```python
from build123d import *

# Parameters (mm, degrees)
BOSS_EXTRUDE1_DEPTH = 3.5
SKETCH2_R           = 3.55
BOSS_EXTRUDE2_DEPTH = 1
SKETCH3_W           = 2.85
SKETCH3_H           = 2.85
BOSS_EXTRUDE3_DEPTH = 1
SKETCH4_W           = 3.9
SKETCH4_H           = 3.9
SKETCH4_R           = 1
BOSS_EXTRUDE4_DEPTH = 2.15
SKETCH5_W           = 1
SKETCH5_H           = 1.5
BOSS_EXTRUDE5_DEPTH = 0.4


with BuildPart() as part:
    # Sketch1 → Boss-Extrude1 (new body)
    with BuildSketch(Plane(origin=(0, 0, 0), x_dir=(1, 0, 0), z_dir=(0, 1, 0))):
        with BuildLine():
            Line((-5, -6), (5, -6))
            ThreePointArc((5, -6), (5.707106781, -5.707106781), (6, -5))
            Line((6, -5), (6, 5))
            ThreePointArc((6, 5), (5.707106781, 5.707106781), (5, 6))
            Line((5, 6), (-5, 6))
            ThreePointArc((-5, 6), (-5.707106781, 5.707106781), (-6, 5))
            Line((-6, 5), (-6, -5))
            ThreePointArc((-6, -5), (-5.707106781, -5.707106781), (-5, -6))
        make_face()
    extrude(amount=BOSS_EXTRUDE1_DEPTH)

    # Sketch2 → Boss-Extrude2 (add)
    with BuildSketch(Plane(origin=(0, 3.5, 0), x_dir=(1, 0, 0), z_dir=(0, 1, 0))):
        with Locations(Location((0, 0, 0), (0, 0, 270))):
            Circle(SKETCH2_R)
    extrude(amount=BOSS_EXTRUDE2_DEPTH)

    # Sketch3 → Boss-Extrude3 (add)
    with BuildSketch(Plane(origin=(0, 4.5, 0), x_dir=(1, 0, 0), z_dir=(0, 1, 0))):
        Rectangle(SKETCH3_W, SKETCH3_H)
    extrude(amount=BOSS_EXTRUDE3_DEPTH)

    # Sketch4 → Boss-Extrude4 (add)
    with BuildSketch(Plane(origin=(0, 5.5, 0), x_dir=(1, 0, 0), z_dir=(0, 1, 0))):
        Rectangle(SKETCH4_W, SKETCH4_H)
        with Locations(Location((0, 0, 0), (0, 0, 90))):
            Circle(SKETCH4_R, mode=Mode.SUBTRACT)
    extrude(amount=BOSS_EXTRUDE4_DEPTH)

    # Sketch5 → Boss-Extrude5 (add)
    with BuildSketch(Plane.XY.offset(6)):
        with Locations((-2.547676789, 0)):
            Rectangle(SKETCH5_W, SKETCH5_H)
        with Locations((2.547676789, 0)):
            Rectangle(SKETCH5_W, SKETCH5_H)
    boss_extrude5 = extrude(amount=BOSS_EXTRUDE5_DEPTH)

    # Mirror1: Boss-Extrude5 across plane
    add(boss_extrude5.mirror(Plane.XY))


solid = part.part
```
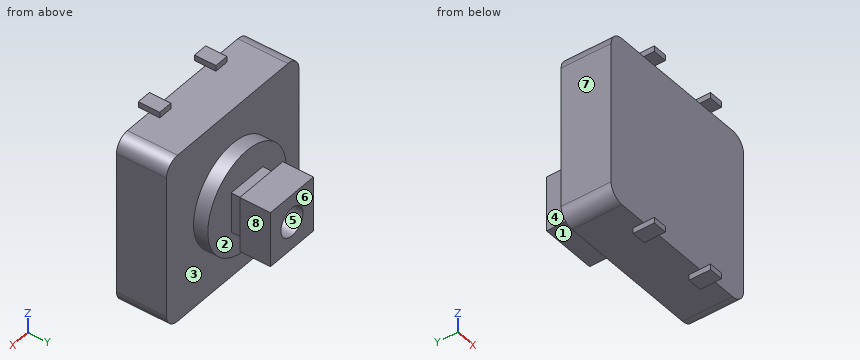
The model under review builds one solid part; all positions refer to its coordinate system, in mm. Face numbers are marked on the shaded views. A direction names the side the tool comes from. Give positions to 0.01 mm unless a question says otherwise; leave off trailing zeros. Write each loop counter-clockwise with the first axis right and the second up, starting at its lowest first coordinate (ties: lowest second). Pieces come first, ordered by that corner, then holes.
(1) Consider section A-A, the plane x = 0. Give the boundary of the cut face in (y, z) (3 decimals), and give its area (3 significant figures).
(2) Consider section D-D, the plane y = 5. Give the boundary of the cut face in (x, z) (3 decimals).
(3) Consider section B-B, the plane y = 3.25. Give the boundary of the cut face in (x, z).
(4) Consider section C-C, the plane z = 0. Give the boundary of the cut face in (x, y) (3 decimals), and give its area (3 significant figures).
(5) To check wall thickness, follow L1, parallel to X at y = 6.95, z = 0; L2, parallel to Y at x = -2, z = 3.25; L3, parallel to Z at x = 4, y = 0.5. State the ranges of each line that lie inside material, in increasing order.
(6) Tool access review of the marked faces 1, 2, 3 and 4: name each direction out of +Z, -Z, +X, -X, +Y, -Y from which nothing blocks a thin tool from reaching the whole face with its end or side.
(7) For P1, Ø0.8, axis at x = -0.5, y = 5, coming from the +Z side (3 decimals); P2, Ø1.7, axis at x = 0, y = 6.5, coming from the -Z side; P3, Ø0.6, axis at x = -0.5, y = 6, coming from the +Z side, all flat-tipped, find the tip position at first contact; note any pin that passes through.
(8) The part is to be moulded in two halves that separate along X. For the marked faces 5, 6, 7 and 8, say which applies: released by +X, released by -X, zero draft, split by the parting line, or undercut.
Returned:
1. outline: (0, -6) - (3.5, -6) - (3.5, -3.55) - (4.5, -3.55) - (4.5, -1.425) - (5.5, -1.425) - (5.5, -1.95) - (7.65, -1.95) - (7.65, -1) - (5.5, -1) - (5.5, 1) - (7.65, 1) - (7.65, 1.95) - (5.5, 1.95) - (5.5, 1.425) - (4.5, 1.425) - (4.5, 3.55) - (3.5, 3.55) - (3.5, 6) - (0, 6) - close
1. area: 56.0 mm2
2. outline: (-1.425, -1.425) - (1.425, -1.425) - (1.425, 1.425) - (-1.425, 1.425) - close
3. outline: (-6, -5) arc R1 ccw to (-5, -6) - (5, -6) arc R1 ccw to (6, -5) - (6, 5) arc R1 ccw to (5, 6) - (-5, 6) arc R1 ccw to (-6, 5) - close
4. outline: (-6, 0) - (6, 0) - (6, 3.5) - (3.55, 3.5) - (3.55, 4.5) - (1.425, 4.5) - (1.425, 5.5) - (1.95, 5.5) - (1.95, 7.65) - (1, 7.65) - (1, 5.5) - (-1, 5.5) - (-1, 7.65) - (-1.95, 7.65) - (-1.95, 5.5) - (-1.425, 5.5) - (-1.425, 4.5) - (-3.55, 4.5) - (-3.55, 3.5) - (-6, 3.5) - close
4. area: 56.0 mm2
5. L1: x = -1.95 to -1, 1 to 1.95
5. L2: y = 0 to 3.5
5. L3: z = -6 to 6
6. face 1: -Z, +X, -X, +Y
6. face 2: none
6. face 3: +Y
6. face 4: +Z, -Z, -X, +Y
7. P1: stops at z = 1.425
7. P2: stops at z = -1.95
7. P3: stops at z = 1.95
8. face 5: undercut
8. face 6: zero draft
8. face 7: released by -X
8. face 8: released by +X
